The model under review builds one solid part; all positions refer to its coordinate system, in mm. A direction names the side the tool comes from. Round coordinates to 2 decimals unless told otherwise and drop trailing zeros. Write each loop counter-clockwise with the first axis right and the second up, starting at its lowest first coordinate (ties: lowest second). Pieces come first, ordered by that corner, then holes. Notation, with made-up numbers: (31, 4.25) - (77, 4.25) arc R21 ccw to (77, 42.25) - close; hole circle Ø6 at (-18.5, -13.5). An arc over 180 degrees is marked (long way). Write each question's results on one line, items separated by ' | '.
```python
from build123d import *

# Parameters (mm, degrees)
BOSS_EXTRUDE1_DEPTH = 37
SKETCH2_W           = 26
SKETCH2_H           = 27
CUT_EXTRUDE2_DEPTH  = 15.3
SKETCH3_W           = 5
SKETCH3_H           = 5
BOSS_EXTRUDE2_DEPTH = 13.8
FILLET1_R           = 0.5
FILLET2_R           = 3
SKETCH4_W           = 13.8
SKETCH4_H           = 16
CUT_EXTRUDE3_DEPTH  = 1
FILLET3_R           = 1
FILLET4_R           = 3


with BuildPart() as part:
    # Sketch1 → Boss-Extrude1 (new body)
    with BuildSketch(Plane.XY):
        Polygon((-8, -16.5), (-9.3, -16.5), (-9.3, -15.4), (-8, -15.4), (-8, 16.5), (8, 16.5), (8, -15.4), (9.3, -15.4), (9.3, -16.5), (8, -16.5), align=None)
    extrude(amount=BOSS_EXTRUDE1_DEPTH)

    # Sketch2 → Cut-Extrude2 (cut)
    with BuildSketch(Plane.ZY.offset(-8)):
        with Locations((18, 1)):
            Rectangle(SKETCH2_W, SKETCH2_H)
    extrude(amount=CUT_EXTRUDE2_DEPTH, mode=Mode.SUBTRACT)

    # Sketch3 → Boss-Extrude2 (add)
    with BuildSketch(Plane(origin=(-7.3, 0, 0), x_dir=(0, 0, -1), z_dir=(1, 0, 0))):
        with Locations((-28.5, 12)):
            Rectangle(SKETCH3_W, SKETCH3_H)
        with Locations((-7.5, 12)):
            Rectangle(SKETCH3_W, SKETCH3_H)
        with Locations((-7.5, -10)):
            Rectangle(SKETCH3_W, SKETCH3_H)
        with Locations((-28.5, -10)):
            Rectangle(SKETCH3_W, SKETCH3_H)
    extrude(amount=BOSS_EXTRUDE2_DEPTH)

    # Fillet1
    fillet1_edges = [part.edges().sort_by_distance(p)[0] for p in [
        (-0.4, 9.5, 31),
        (-0.4, 9.5, 5),
        (-0.4, -7.5, 31),
        (-0.4, -12.5, 26),
        (-0.4, -7.5, 5),
        (-0.4, -12.5, 10),
    ]]
    fillet(fillet1_edges, radius=FILLET1_R)

    # Fillet2
    fillet2_edges = [part.edges().sort_by_distance(p)[0] for p in [
        (-0.4, 9.5, 26),
        (-0.4, 9.5, 10),
        (-0.4, -7.5, 26),
        (-0.4, -7.5, 10),
    ]]
    fillet(fillet2_edges, radius=FILLET2_R)

    # Sketch4 → Cut-Extrude3 (cut)
    with BuildSketch(Plane.XZ.offset(-14.5)):
        with Locations((-0.4, 18)):
            Rectangle(SKETCH4_W, SKETCH4_H)
    extrude(amount=-CUT_EXTRUDE3_DEPTH, mode=Mode.SUBTRACT)

    # Fillet3
    fillet3_edges = [part.edges().sort_by_distance(p)[0] for p in [
        (-0.4, 15.5, 10),
        (-0.4, 15.5, 26),
    ]]
    fillet(fillet3_edges, radius=FILLET3_R)

    # Fillet4
    fillet4_edges = [part.edges().sort_by_distance(p)[0] for p in [
        (0, 16.5, 0),
        (0, 16.5, 37),
    ]]
    fillet(fillet4_edges, radius=FILLET4_R)


solid = part.part
```
Q1. We need section D-D (z = 6.5). State the section outline as (x, y) points, plus the area to 3 significant figures.
Evaluation:
outline: (-9.3, -16.5) - (9.3, -16.5) - (9.3, -15.4) - (8, -15.4) - (8, -12.5) - (6.5, -12.5) - (6.5, -7.5) - (-7.3, -7.5) - (-7.3, 9.5) - (6.5, 9.5) - (6.5, 14.5) - (8, 14.5) - (8, 16.5) - (-8, 16.5) - (-8, -15.4) - (-9.3, -15.4) - close | area: 256 mm^2
Q2. We need section B-B (y = 6.5). State the section outline as (x, z) points, plus the area to 3 significant figures.
Evaluation:
outline: (-8, 0) - (8, 0) - (8, 5) - (-7.3, 5) - (-7.3, 31) - (8, 31) - (8, 37) - (-8, 37) - close | area: 194 mm^2
Q3. For probe 1 along Y at (x, z) = (-1, 17); probe 2 along Y at (x, z) = (3.5, 30); probe 3 along Z at (x, y) = (-3.5, 5.5), list the stretches that pass through material, from the lowest coordinate up.
Evaluation:
probe 1: y = -16.5 to -12.5, 15.5 to 16.5 | probe 2: y = -16.5 to -7.5, 9.5 to 16.5 | probe 3: z = 0 to 5, 31 to 37
Q4. We need section C-C (z = 19.5). State the section outline as (x, y) points, plus the area to 3 significant figures.
Evaluation:
outline: (-9.3, -16.5) - (9.3, -16.5) - (9.3, -15.4) - (8, -15.4) - (8, -12.5) - (-7.3, -12.5) - (-7.3, 15.5) - (6.5, 15.5) - (6.5, 14.5) - (8, 14.5) - (8, 16.5) - (-8, 16.5) - (-8, -15.4) - (-9.3, -15.4) - close | area: 104 mm^2
Q5. The part is to be moulded in two halves that separate along Y. For faces 1 (the flat face through (0, 9.5, 30)), 2 (the flat face through (0, 16.5, 18)), 3 (the flat face through (8, 15, 18)), 4 (the flat face through (0, -7.5, 6)), say which applies: released by +Y, released by -Y, zero draft, split by the parting line, or undercut.
Evaluation:
face 1: undercut | face 2: released by +Y | face 3: zero draft | face 4: undercut
Q6. Insertion check: P1, Ø0.5, axis at y = 15, z = 17.5, coming from the -X side; P2, Ø3, axis at y = 1.5, z = 10, coming from the +X side; P3, Ø1.5, axis at y = 12.5, z = 29, coming from the +X side. Each pin has a flat end and moves straight along its axis. Give the tip position at first contact, or say it passes through.
Evaluation:
P1: stops at x = -8 | P2: stops at x = -7.3 | P3: stops at x = 6.5
Q7. Tool access review of faces 5 (the flat face through (6.5, -10, 29)), 6 (the flat face through (-9, -15.4, 18)), 7 (the flat face through (0, -16.5, 18)), 8 (the cylindrical face through (-0.303, 15.215, 25.699)), 9 (the cylindrical face through (0.11, 15.64, 0.9)): name each direction out of +Z, -Z, +X, -X, +Y, -Y from which nothing blocks a thin tool from reaching the whole face with its end or side.
Evaluation:
face 5: +X | face 6: +Z, -Z, -X, +Y | face 7: +Z, -Z, +X, -X, -Y | face 8: none | face 9: -Z, +X, -X, +Y
